The model under review builds one solid part; all positions refer to its coordinate system, in mm. A direction names the side the tool comes from. Round coordinates to 2 decimals unless told otherwise and drop trailing zeros. Order: outer loops, then holes, each group sorted by start corner. A loop starts at its lowest first (then second) coordinate and runs counter-clockwise, first axis right, second up. Notation, with made-up numbers: M 85.5,27 L 142.5,27 A23 cw 142.5,58 Z; hole C 30,-39 d8. An arc over 180 degrees is marked long. Use a Markdown table: item, result. Add a question column.
1. To check wall thickness, follow probe 1 along Y at (x, z) = (11.55, 0); probe 2 along Y at (x, z) = (14.25, 0); probe 3 along Z at (x, y) = (14.5, 1.75). State the ranges of each line that lie inside material, in increasing order.
2. Consider section B-B on x = 16.25. State the section outline as (y, z) points, then the cut area to 3 significant figures.
3. The part is to be moulded in two halves that separate along Y. For faces 6 (the flat face through (22.03, -6, -10)), 7 (the flat face through (20.798, 5.83, -9.913)), 8 (the conical face through (8.5, 6.23, 1.96)), say which applies: +Y half, -Y half, draft (parallel to the pull), parting line (faces both ways), or undercut.
4. Insertion check: P1, Ø3, axis at x = 20.5, z = 1, coming from the +Y side; P2, Ø1.7, axis at y = -7.5, z = 7, coming from the +X side; P3, Ø4, axis at x = 8, z = 0, coming from the +Y side; P4, Ø3, axis at y = -8, z = -6.5, coming from the +X side. Each pin has a flat end and moves straight along its axis. Give the tip position at first contact, or say it passes through.
5. For faces 1 (the cylindrical face through (11.04, -1.22, -0.27)), 2 (the conical face through (4.469, 8.416, 9.177)), 3 (the flat face through (8, -1.75, 0)), 4 (the flat face through (22.03, 6, 10)), 5 (the flat face through (20.798, -5.67, -10.006)), list the 3-axis set-ups (+Z, -Z, +X, -X, +Y, -Y) from which the entire face can be reached by the end or side of a thin tool; tool diameter is ignored.
6. Consider section A-A on x = 20. State the section outline as (y, z) points, then the cut area to 3 significant figures.
from build123d import *

# Parameters (mm, degrees)
SKETCH1_R           = 13.75
BOSS_EXTRUDE1_DEPTH = 22.03
SKETCH3_W           = 3.5
SKETCH3_H           = 3.5
CUT_EXTRUDE1_DEPTH  = 3.75
CUT_EXTRUDE2_START  = -12
CUT_EXTRUDE2_DEPTH  = 2.5
CUT_EXTRUDE4_START  = -9.5
SKETCH4_29_R        = 11.5
CUT_EXTRUDE4_DEPTH  = 7.5
CUT_EXTRUDE5_START  = -2
SKETCH4_30_R        = 1.25
CUT_EXTRUDE5_DEPTH  = 2
CHAMFER1_SIZE       = 1.5
CHAMFER2_SIZE       = 1.5
CHAMFER2_SIZE_2     = 2.841585372


# Read off the part's stored shape, not the designer's step: Cut-Revolve-Thin1
with BuildPart() as part:
    # Sketch1 → Boss-Extrude1 (new body)
    with BuildSketch(Plane(origin=(0, 0, 0), x_dir=(0, 0, -1), z_dir=(1, 0, 0))):
        Circle(SKETCH1_R)
    extrude(amount=BOSS_EXTRUDE1_DEPTH)

    # Sketch2 → Cut-Revolve1 (revolve, cut)
    with BuildSketch(Plane(origin=(46.159172163, 0, 11.54266395), x_dir=(0, 0, 1), z_dir=(0, 1, 0)), mode=Mode.PRIVATE) as cut_revolve1_sk:
        with BuildLine():
            Line((-22.29266395, -43.379172163), (-21.047307804, -43.379172163))
            Line((-21.047307804, -43.379172163), (-21.047307804, -42.629172163))
            ThreePointArc((-21.047307804, -42.629172163), (-20.923021734, -42.215672371), (-20.591355596, -41.939218617))
            Line((-20.591355596, -41.939218617), (-15.75766395, -39.879172163))
            Line((-15.75766395, -39.879172163), (-11.54266395, -39.879172163))
            Line((-11.54266395, -39.879172163), (-11.54266395, -46.159172163))
            Line((-11.54266395, -46.159172163), (-23.04266395, -46.159172163))
            Line((-23.04266395, -46.159172163), (-23.04266395, -44.129172163))
            ThreePointArc((-23.04266395, -44.129172163), (-22.822994036, -43.598842077), (-22.29266395, -43.379172163))
        make_face()
    revolve(cut_revolve1_sk.sketch.rotate(Axis((-993.090827837, 0, 0), (1, 0, 0)), 180), axis=Axis((-993.090827837, 0, 0), (1, 0, 0)), mode=Mode.SUBTRACT)

    # Sketch3 → Cut-Extrude1 (cut)
    with BuildSketch(Plane.ZY.offset(-6.28)):
        Rectangle(SKETCH3_W, SKETCH3_H)
    extrude(amount=-CUT_EXTRUDE1_DEPTH, mode=Mode.SUBTRACT)

    # Sketch4 → Cut-Extrude2 (cut)
    with BuildSketch(Plane(origin=(10.03, 32, 0), x_dir=(0, 0, 1), z_dir=(-1, 0, 0)).offset(CUT_EXTRUDE2_START)):
        Polygon((-6.639528096, -20.5), (-13.279056191, -32), (-6.639528096, -43.5), (6.639528096, -43.5), (13.279056191, -32), (6.639528096, -20.5), align=None)
    extrude(amount=CUT_EXTRUDE2_DEPTH, mode=Mode.SUBTRACT)

    # Sketch4<29> → Cut-Extrude4 (cut)
    with BuildSketch(Plane(origin=(10.03, 32, 0), x_dir=(0, 0, 1), z_dir=(-1, 0, 0)).offset(CUT_EXTRUDE4_START)):
        with Locations((0, -32)):
            Circle(SKETCH4_29_R)
    extrude(amount=CUT_EXTRUDE4_DEPTH, mode=Mode.SUBTRACT)

    # Sketch4<30> → Cut-Extrude5 (cut)
    with BuildSketch(Plane(origin=(10.03, 32, 0), x_dir=(0, 0, 1), z_dir=(-1, 0, 0)).offset(CUT_EXTRUDE5_START)):
        with Locations((0, -32)):
            Circle(SKETCH4_30_R)
    extrude(amount=CUT_EXTRUDE5_DEPTH, mode=Mode.SUBTRACT)

    # Cut-Revolve-Thin1 outline → Cut-Revolve-Thin1 (revolve, cut)
    with BuildSketch(Plane.YX):
        Polygon((13.75, 10.03), (6.25, 10.03), (6.25, 7.28), (13.75, 4.083613153), align=None)
    revolve(axis=Axis((0, 0, 0), (1, 0, 0)), mode=Mode.SUBTRACT)

    # Chamfer1
    # the kernel refuses this chamfer: 1.5 mm, written as the material it adds along each edge
    with BuildSketch(Plane(origin=(10.03, 0, 0), x_dir=(0, 1, 0), z_dir=(0, 0, -1))) as chamfer1_piece_1:
        Polygon((6.25, -CHAMFER1_SIZE), (6.25 + CHAMFER1_SIZE, 0), (6.25, 0), align=None)
    revolve(axis=Axis((10.03, 0, 0), (1, 0, 0)))
    # the kernel refuses this chamfer: 1.5 mm, written as the material it takes off along each edge
    with BuildSketch(Plane(origin=(0, 0, 0), x_dir=(0, 0, -1), z_dir=(0, -1, 0))) as chamfer1_2_piece_1:
        Polygon((13.75, CHAMFER1_SIZE), (13.75 - CHAMFER1_SIZE, 0), (13.75, 0), align=None)
    revolve(axis=Axis((0, 0, 0), (1, 0, 0)), mode=Mode.SUBTRACT)
    with BuildSketch(Plane(origin=(22.03, 0, 0), x_dir=(0, 0, -1), z_dir=(0, -1, 0))) as chamfer1_2_piece_2:
        Polygon((13.75, -CHAMFER1_SIZE), (13.75 - CHAMFER1_SIZE, 0), (13.75, 0), align=None)
    revolve(axis=Axis((22.03, 0, 0), (1, 0, 0)), mode=Mode.SUBTRACT)
    with BuildSketch(Plane(origin=(10.03, 0, 0), x_dir=(0, 0, -1), z_dir=(0, 1, 0))) as chamfer1_2_piece_3:
        Polygon((13.75 - CHAMFER1_SIZE, 0), (13.75, -CHAMFER1_SIZE), (13.75, 0), align=None)
    revolve(axis=Axis((10.03, 0, 0), (-1, 0, 0)), mode=Mode.SUBTRACT)

    # Chamfer2
    # the kernel refuses this chamfer: 2.841585372, 1.5 mm, written as the material it adds along each edge
    with BuildSketch(Plane(origin=(7.28, 0, 0), x_dir=(0, 1, 0), z_dir=(0, 0, -1))) as chamfer2_piece_1:
        Polygon((6.25, CHAMFER2_SIZE), (6.25 + CHAMFER2_SIZE_2 * 0.919938061778, -CHAMFER2_SIZE_2 * 0.392063722763), (6.25, 0), align=None)
    revolve(axis=Axis((7.28, 0, 0), (1, 0, 0)))
    # the kernel refuses this chamfer: 2.841585372, 1.5 mm, written as the material it takes off along each edge
    with BuildSketch(Plane(origin=(4.083613153, 0, 0), x_dir=(0, 1, 0), z_dir=(0, 0, -1))) as chamfer2_2_piece_1:
        Polygon((13.75 - CHAMFER2_SIZE * 0.919938061679, CHAMFER2_SIZE * 0.392063722721), (13.75, -CHAMFER2_SIZE_2), (13.75, 0), align=None)
    revolve(axis=Axis((4.083613153, 0, 0), (1, 0, 0)), revolution_arc=270, mode=Mode.SUBTRACT)
    with BuildSketch(Plane(origin=(4.083613153, 0, 0), x_dir=(0, 0, -1), z_dir=(0, -1, 0))) as chamfer2_2_piece_2:
        Polygon((13.75 - CHAMFER2_SIZE * 0.919938061679, CHAMFER2_SIZE * 0.392063722721), (13.75, -CHAMFER2_SIZE_2), (13.75, 0), align=None)
    revolve(axis=Axis((4.083613153, 0, 0), (1, 0, 0)), revolution_arc=90, mode=Mode.SUBTRACT)


solid = part.part
Answer block:
| question | item | result |
|---|---|---|
| 1 | probe 1 | -13.75 to -1.25, 1.25 to 13.75 |
| 1 | probe 2 | -13.75 to -11.5, 11.5 to 13.75 |
| 1 | probe 3 | -13.64 to -11.37, 11.37 to 13.64 |
| 2 | outline | C 0,0 d27.5; hole C 0,0 d23 |
| 2 | area | 178 mm^2 |
| 3 | face 6 | draft |
| 3 | face 7 | undercut |
| 3 | face 8 | parting line |
| 4 | P1 | y = 13.75 |
| 4 | P2 | x = 12.03 |
| 4 | P3 | y = 9.25 |
| 4 | P4 | x = 19.53 |
| 5 | face 1 | +X, -X |
| 5 | face 2 | none |
| 5 | face 3 | -X |
| 5 | face 4 | +Z, -Z, +X, +Y, -Y |
| 5 | face 5 | +X |
| 6 | outline | C 0,0 d27.5; hole M -11.5,-6.64 L 0,-13.28 L 11.5,-6.64 L 11.5,6.64 L 0,13.28 L -11.5,6.64 Z |
| 6 | area | 136 mm^2 |
